```python
from build123d import *

# Parameters (mm, degrees)
SQUARE_TUBE_40_X_40_X_4_2_DEPTH = 1700.022


with BuildPart() as part:
    # Sketch13 → Square tube 40 X 40 X 4(2) (new body)
    with BuildSketch(Plane.XY.offset(-850.011)):
        with BuildLine():
            Line((-12, -20), (12, -20))
            ThreePointArc((12, -20), (17.656854249, -17.656854249), (20, -12))
            Line((20, -12), (20, 12))
            ThreePointArc((20, 12), (17.656854249, 17.656854249), (12, 20))
            Line((12, 20), (-12, 20))
            ThreePointArc((-12, 20), (-17.656854249, 17.656854249), (-20, 12))
            Line((-20, 12), (-20, -12))
            ThreePointArc((-20, -12), (-17.656854249, -17.656854249), (-12, -20))
        make_face()
        with BuildLine():
            Line((-12, -16), (12, -16))
            ThreePointArc((12, -16), (14.828427125, -14.828427125), (16, -12))
            Line((16, -12), (16, 12))
            ThreePointArc((16, 12), (14.828427125, 14.828427125), (12, 16))
            Line((12, 16), (-12, 16))
            ThreePointArc((-12, 16), (-14.828427125, 14.828427125), (-16, 12))
            Line((-16, 12), (-16, -12))
            ThreePointArc((-16, -12), (-14.828427125, -14.828427125), (-12, -16))
        make_face(mode=Mode.SUBTRACT)
    extrude(amount=SQUARE_TUBE_40_X_40_X_4_2_DEPTH)


solid = part.part
```
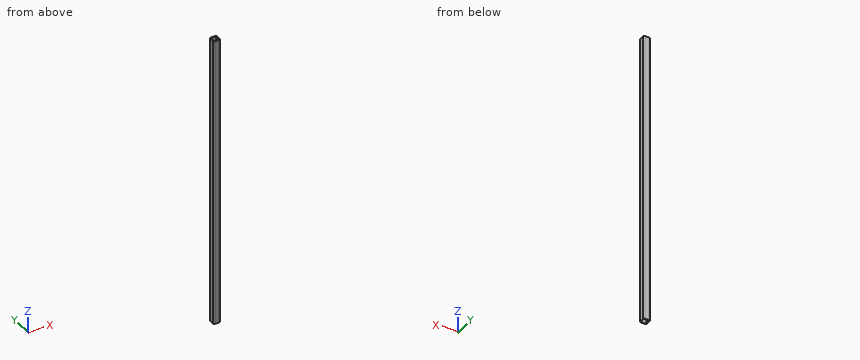
CAD build for the part. Positions are in the model's coordinates, mm. Round coordinates to 2 decimals unless told otherwise and drop trailing zeros. Loops run counter-clockwise (first coordinate to the right, second up) from the corner with the lowest first, then second, coordinate; pieces in that order, holes last. Notation, with made-up numbers: M 11,29 L 43,29 A13 ccw 43,49 Z; hole C 50.5,59.25 d4. An arc over 180 degrees is marked long. Use a Markdown table: item, result. Add a question column.
(1) Cut at A-A (y = 5.5). Give the cut face in (x, z).
(2) Cut at C-C (z = 119). Give the cut face in (x, y).
(3) Drill centre lines: line 1 (Y direction, x = -7, z = 676); line 2 (X direction, y = 13.5, z = 695). Where is each one in solid material? Low to high.
(4) Flat gauge pin, fed straight in: pin 1 (1 mm diameter, centred on x = 14.5, z = 169, fed in from -Y). Where does the tip first touch, or does it go through?
Geometry says:
| question | item | result |
|---|---|---|
| 1 | outline | M -20,-850.01 L -16,-850.01 L -16,850.01 L -20,850.01 Z; M 16,-850.01 L 20,-850.01 L 20,850.01 L 16,850.01 Z |
| 2 | outline | M -20,-12 A8 ccw -12,-20 L 12,-20 A8 ccw 20,-12 L 20,12 A8 ccw 12,20 L -12,20 A8 ccw -20,12 Z; hole M -16,-12 A4 ccw -12,-16 L 12,-16 A4 ccw 16,-12 L 16,12 A4 ccw 12,16 L -12,16 A4 ccw -16,12 Z |
| 3 | line 1 | y = -20 to -16, 16 to 20 |
| 3 | line 2 | x = -19.86 to -15.71, 15.71 to 19.86 |
| 4 | pin 1 | stops at y = -19.75 |
